from build123d import *

# Parameters (mm, degrees)
SKETCH_1_R      = 4
EXTRUDE_1_DEPTH = 5


with BuildPart() as part:
    # 草图1 → 凸台-拉伸1 (new body)
    with BuildSketch(Plane(origin=(0, 0, 0), x_dir=(1, 0, 0), z_dir=(0, 1, 0))):
        with BuildLine():
            Line((-76.197907508, 60.368596958), (-79.079757453, 66.278376643))
            ThreePointArc((-79.079757453, 66.278376643), (-90.335533029, 66.937484633), (-87.619490015, 55.994449518))
            Line((-87.619490015, 55.994449518), (-82.39006252, 53.837347743))
            Line((-82.39006252, 53.837347743), (70.005752496, -90.646269203))
            Line((70.005752496, -90.646269203), (72.438335487, -95.753376015))
            ThreePointArc((72.438335487, -95.753376015), (83.510505182, -97.882687035), (82.252798454, -86.677996903))
            Line((82.252798454, -86.677996903), (76.197907508, -84.115019988))
            Line((76.197907508, -84.115019988), (-76.197907508, 60.368596958))
        make_face()
        with Locations(Location((-84.950212753, 62.465535895, 0), (0, 0, 270))):
            Circle(SKETCH_1_R, mode=Mode.SUBTRACT)
        with Locations(Location((78.758057741, -92.74320814, 0), (0, 0, 270))):
            Circle(SKETCH_1_R, mode=Mode.SUBTRACT)
    extrude(amount=EXTRUDE_1_DEPTH)


solid = part.part
Can you work these out from the model? Positions are in its coordinate system, mm. Coordinates: 2 decimals unless noted, no trailing zeros. Write each loop counter-clockwise with the first axis right and the second up, starting at its lowest first coordinate (ties: lowest second). Pieces come first, ordered by that corner, then holes. Notation, with made-up numbers: (11.25, -32.75) -> (41.25, -32.75) arc R31 ccw to (41.25, 5.25) -> close; hole circle Ø7 at (40, 61.25). An arc over 180 degrees is marked (long way). Write each question's results on one line, items separated by ' | '. Start each with the question number.
Q1. We'd pull the mould along Z, two halves only. Please class faces 1 (the face through (79.268, 2.465, 85.414)), 2 (the face through (-90.216, 2.465, -67.077)), 3 (the face through (78.934, 2.465, 88.747)): +Z half, -Z half, draft (parallel to the pull), parting line (faces both ways), or undercut.
Q2. If I drill on probe 1 along X at (y, z) = (3.4, 3.5); probe 2 along X at (y, z) = (1.85, -10); probe 3 along Z at (x, y) = (15.5, 1.85), over which ranges is the centre line in solid material (lowest first)?
Q3. I'm going to push flat-ended pins straight in: pin 1 (2 mm diameter, centred on x = 58, y = 3.5, fed in from +Z); pin 2 (1.5 mm diameter, centred on y = 3.5, z = -0.5, fed in from -X); pin 3 (3 mm diameter, centred on x = 42.5, y = 4, fed in from +Z). Where does each tip first touch, or does it pass through?
Q4. Imagine slicing it at B-B (x = 56). Write out the boundary of the cut face in (y, z), then the cut area to 3 significant figures.
Q5. Imagine slicing it at C-C (z = 21). Write out the boundary of the cut face in (x, y).
Q6. Imagine slicing it at A-A (y = 1.65). Write out the boundary of the cut face in (x, z).
Taken from the geometry:
1) face 1: -Z half | face 2: parting line | face 3: undercut
2) probe 1: x = -21.91 to -8.83 | probe 2: x = -36.15 to -23.07 | probe 3: z = 26.57 to 38.97
3) pin 1: stops at z = 80.21 | pin 2: stops at x = -26.92 | pin 3: stops at z = 65.99
4) outline: (0, 64.97) -> (5, 64.97) -> (5, 77.37) -> (0, 77.37) -> close | area: 62.0 mm^2
5) outline: (-3.45, 0) -> (9.63, 0) -> (9.63, 5) -> (-3.45, 5) -> close
6) outline: (-87.62, -55.99) arc R7 ccw (long way) to (-79.08, -66.28) -> (-76.2, -60.37) -> (76.2, 84.12) -> (82.25, 86.68) arc R7 ccw (long way) to (72.44, 95.75) -> (70.01, 90.65) -> (-82.39, -53.84) -> close; hole circle Ø8 at (-84.95, -62.47); hole circle Ø8 at (78.76, 92.74)
